from build123d import *

# Parameters (mm, degrees)
SKETCH_W        = 119.87
SKETCH_H        = 77.81
SKETCH_R        = 1.45
PAD_DEPTH       = 5
SKETCH045_R     = 2.5
PAD032_DEPTH    = 5
SKETCH046_R     = 2.3
POCKET_DEPTH    = 3.5
SKETCH051_W     = 99.87
SKETCH051_H     = 67.81
POCKET012_DEPTH = 2
FILLET001_R     = 3


with BuildPart() as part:
    # Sketch → Pad (new body)
    with BuildSketch(Plane.XY):
        with Locations((56.935, -32.905)):
            Rectangle(SKETCH_W, SKETCH_H)
        with Locations((0, -68.81)):
            Circle(SKETCH_R, mode=Mode.SUBTRACT)
        with Locations((113.57, -68.81)):
            Circle(SKETCH_R, mode=Mode.SUBTRACT)
        with Locations((113.57, 2.7)):
            Circle(SKETCH_R, mode=Mode.SUBTRACT)
        with Locations((0, 2.7)):
            Circle(SKETCH_R, mode=Mode.SUBTRACT)
    extrude(amount=PAD_DEPTH)

    # Sketch045 (on Face9 of Pad) → Pad032 (join)
    with BuildSketch(Plane(origin=(0, 0, 0), x_dir=(1, 0, 0), z_dir=(0, 0, -1))):
        with BuildLine():
            ThreePointArc((-9.566038, 63.821132), (-15, 58.84), (-9.566038, 53.858868))
            ThreePointArc((-3, 47.84), (-4.959164, 52.29364), (-9.566038, 53.858868))
            Line((-3, 69.84), (-3, 47.84))
            ThreePointArc((-9.566038, 63.821132), (-4.959164, 65.38636), (-3, 69.84))
        make_face()
        with Locations((-10, 58.84)):
            Circle(SKETCH045_R, mode=Mode.SUBTRACT)
        with BuildLine():
            ThreePointArc((-9.566038, 11.951132), (-15, 6.97), (-9.566038, 1.988868))
            ThreePointArc((-3, -4.03), (-4.959164, 0.42364), (-9.566038, 1.988868))
            Line((-3, 17.97), (-3, -4.03))
            ThreePointArc((-9.566038, 11.951132), (-4.959164, 13.51636), (-3, 17.97))
        make_face()
        with Locations((-10, 6.97)):
            Circle(SKETCH045_R, mode=Mode.SUBTRACT)
        with BuildLine():
            ThreePointArc((123.436038, 1.988868), (128.87, 6.97), (123.436038, 11.951132))
            ThreePointArc((116.87, 17.97), (118.829164, 13.51636), (123.436038, 11.951132))
            Line((116.87, 17.97), (116.87, -4.03))
            ThreePointArc((123.436038, 1.988868), (118.829164, 0.42364), (116.87, -4.03))
        make_face()
        with Locations((123.87, 6.97)):
            Circle(SKETCH045_R, mode=Mode.SUBTRACT)
        with BuildLine():
            ThreePointArc((123.436038, 53.858868), (128.87, 58.84), (123.436038, 63.821132))
            ThreePointArc((116.87, 69.84), (118.829164, 65.38636), (123.436038, 63.821132))
            Line((116.87, 69.84), (116.87, 47.84))
            ThreePointArc((123.436038, 53.858868), (118.829164, 52.29364), (116.87, 47.84))
        make_face()
        with Locations((123.87, 58.84)):
            Circle(SKETCH045_R, mode=Mode.SUBTRACT)
    extrude(amount=-PAD032_DEPTH)

    # Sketch046 (on Face21 of Pad032) → Pocket (cut)
    with BuildSketch(Plane(origin=(0, 0, 0), x_dir=(1, 0, 0), z_dir=(0, 0, -1))):
        with Locations((0, -2.7)):
            Circle(SKETCH046_R)
        with Locations((113.57, -2.7)):
            Circle(SKETCH046_R)
        with Locations((113.57, 68.81)):
            Circle(SKETCH046_R)
        with Locations((0, 68.81)):
            Circle(SKETCH046_R)
    extrude(amount=-POCKET_DEPTH, mode=Mode.SUBTRACT)

    # Sketch051 (on Face4 of Pocket) → Pocket012 (cut)
    with BuildSketch(Plane.XY.offset(5)):
        with Locations((56.935, -32.905)):
            Rectangle(SKETCH051_W, SKETCH051_H)
    extrude(amount=-POCKET012_DEPTH, mode=Mode.SUBTRACT)

    # Fillet001
    fillet001_edges = [part.edges().sort_by_distance(p)[0] for p in [
        (116.87, -71.81, 2.5),
        (-3, -71.81, 2.5),
        (-3, 6, 2.5),
        (116.87, 6, 2.5),
    ]]
    fillet(fillet001_edges, radius=FILLET001_R)


with BuildPart() as part_1:
    # Body placement: moved
    add(part.part.moved(Location((0, 0, -12.73))))


solid = part_1.part
Work out the finished part from the listing and answer in its coordinate system (mm). A direction names the side the tool comes from. Give positions to 0.01 mm unless a question says otherwise; leave off trailing zeros. Order: outer loops, then holes, each group sorted by start corner. A loop starts at its lowest first (then second) coordinate and runs counter-clockwise, first axis right, second up. Notation, with made-up numbers: (83, 41.5) - (129, 41.5) arc R26 cw to (129, 66.5) - close; hole circle Ø7 at (12.5, -9). An arc over 180 degrees is marked (long way). Answer as CSV lines item,"result". Start each with the question number.
Q1. The mould has two halves that part along X. Classify faces 1 (the face through (0.669, -70.096, -8.49)), 2 (the face through (116.87, -33, -10)), 3 (the face through (-3, -33, -10)): +X half, -X half, draft (parallel to the pull), parting line (faces both ways), or undercut.
Q2. For faces 4 (the face through (121.886, -5.449, -10.265)), 5 (the face through (115.1, 3.2, -9.23)), determine the directions among +Z, -Z, +X, -X, +Y, -Y from which every point of the face is accessible in a straight line to the end or side of a thin tool.
Q3. The part is cut by section D-D (z = -10.65). Give the number of separate pieces and of enclosed holes in the cut face, then the cut area to 3 significant figures.
Q4. The part is cut by section B-B (x = 95.5). Write down the section's boundary in (y, z).
Q5. The part is cut by section C-C (y = -15). Write down the section's boundary in (x, z).
Q6. Given pin 1 Ø1 at (x, y) = (45.5, -15) entering from +Z; pin 2 Ø2 at (y, z) = (-35.5, -12) entering from +X; pin 3 Ø5 at (x, y) = (0, -68) entering from -Z; pin 4 Ø3.5 at (x, y) = (113.57, -68.81) entering from -Z, each flat-ended and moving along its own axis, determine where each tip first touches the part or whether it passes through.
Q7. Find the intervals of material crossed by L1, parallel to Y at x = 0, z = -11.3; L2, parallel to X at y = -58.84, z = -10.4; L3, parallel to Y at x = 123.87, z = -10.95, in increasing order. Write a range as [from, to].
Q8. The part is cut by section A-A (y = -58.84). Write down the section's boundary in (x, z), then the cut area to 3 significant figures.
Check result:
1,face 1,"undercut"
1,face 2,"+X half"
1,face 3,"-X half"
2,face 4,"+Z, -Z"
2,face 5,"-Z"
3,separate pieces,"1"
3,enclosed holes,"8"
3,area,"9,670 mm²"
4,outline,"(-71.81, -12.73) - (6, -12.73) - (6, -7.73) - (1, -7.73) - (1, -9.73) - (-66.81, -9.73) - (-66.81, -7.73) - (-71.81, -7.73) - close"
5,outline,"(-3.78, -12.73) - (117.65, -12.73) - (117.65, -7.73) - (106.87, -7.73) - (106.87, -9.73) - (7, -9.73) - (7, -7.73) - (-3.78, -7.73) - close"
6,pin 1,"stops at z = -9.73"
6,pin 2,"stops at x = 116.87"
6,pin 3,"stops at z = -12.73"
6,pin 4,"stops at z = -9.23"
7,L1,"y = [-71.81, -71.11], [-66.51, 0.4], [5, 6]"
7,L2,"x = [-15, -12.5], [-7.5, 121.37], [126.37, 128.87]"
7,L3,"y = [-63.84, -61.34], [-56.34, -53.84], [-11.97, -9.47], [-4.47, -1.97]"
8,outline,"(-15, -12.73) - (-12.5, -12.73) - (-12.5, -7.73) - (-15, -7.73) - close; (-7.5, -12.73) - (121.37, -12.73) - (121.37, -7.73) - (106.87, -7.73) - (106.87, -9.73) - (7, -9.73) - (7, -7.73) - (-7.5, -7.73) - close; (126.37, -12.73) - (128.87, -12.73) - (128.87, -7.73) - (126.37, -7.73) - close"
8,area,"470 mm²"
